Autodesk Inventor part; units mm, degrees
ref_plane "YZ Plane" through (0, 0, 0) normal (1, 0, 0) x (0, 1, 0)
ref_plane "XZ Plane" through (0, 0, 0) normal (0, 1, 0) x (-1, 0, 0)
ref_plane "XY Plane" through (0, 0, 0) normal (0, 0, 1) x (1, 0, 0)
sketch "스케치1" plane through (0, 0, 0) normal (0, 0, 1) x (1, 0, 0)
  line L0 (15, -15) -> (-15, -15)
  line L1 (-15, -15) -> (-15, 15)
  line L2 (-15, 15) -> (15, 15)
  line L3 (15, 15) -> (15, -15)
  line L4 (15, -15) -> (-15, 15) construction
  line L5 (-15, -15) -> (15, 15) construction
  point P0 (0, 0)
  dimension "d0" = 30
  dimension "d1" = 30
extrude "돌출1" add sketch "스케치1" along normal blind 2
sketch "스케치2" plane through (0, 0, 2) normal (0, 0, 1) x (1, 0, 0)
  line L0 (-15, 15) -> (-15, -15)
  line L1 (-15, -15) -> (15, -15)
  line L2 (-15, 15) -> (-12, 15)
  line L3 (-12, 15) -> (-12, -15)
  line L4 (-12, -15) -> (-15, -15)
  line L5 (-15, -15) -> (-15, 15)
  line L6 (15, -15) -> (15, 15)
  line L7 (15, 15) -> (12, 15)
  line L8 (12, 15) -> (12, -15)
  line L9 (12, -15) -> (15, -15)
  line L10 (15, -15) -> (15, 15)
  point P0 (0, 0)
  dimension "d4" = 3
  dimension "d5" = 3
extrude "돌출2" add sketch "스케치2" along normal blind 30
sketch "스케치3" plane through (0, 0, 0) normal (0, 0, -1) x (-1, 0, 0)
  circle A0 centre (0, 0) radius 5
  dimension "d8" = 10
extrude "돌출3" add sketch "스케치3" along normal blind 1
sketch "스케치4" plane through (15, -15, 0) normal (1, 0, 0) x (0, 0, -1)
  line L0 (0, 0) -> (-39, 0)
  line L1 (-39, 0) -> (-26.5, 0)
  line L2 (-2, 0) -> (-32, 0)
  line L3 (-26.5, 0) -> (-26.5, 10)
  circle A0 centre (-26.5, 10) radius 2.5
  line L4 (0, 0) -> (-32, 0)
  line L5 (0, 0) -> (-34, 0)
  line L6 (-34, 0) -> (-21.5, 0)
  line L7 (-21.5, 0) -> (-21.5, 10)
  circle A1 centre (-21.5, 10) radius 2.5
  point P0 (0, 15)
  dimension "d11" = 39
  dimension "d12" = 12.5
  dimension "d13" = 5
  dimension "d14" = 10
  dimension "d32" = 34
  dimension "d33" = 12.5
extrude "돌출4" add sketch "스케치4" against normal blind 12.5 contours A1
sketch "스케치5" plane through (-15, -15, 0) normal (-1, 0, 0) x (0, 0, 1)
  circle A0 centre (26.5, 10) radius 2.5
  circle A1 centre (21.5, 10) radius 2.5
  circle A2 centre (21.5, 10) radius 2.5
  point P0 (0, 15)
extrude "돌출5" add sketch "스케치5" against normal blind 12.5 contours A1
sketch "스케치6" plane through (15, -15, 0) normal (1, 0, 0) x (0, 0, -1)
  line L0 (0, 30) -> (-32, 30)
  line L1 (-2, 30) -> (-32, 30)
  line L2 (-2, 30) -> (-32, 30)
  line L3 (0, 30) -> (-32, 30)
  line L4 (-2, 0) -> (-2, 30)
  line L5 (-2, 30) -> (-2, 0)
  line L6 (0, 30) -> (-32, 30)
  line L7 (-2, 30) -> (-2, 0)
  line L8 (0, 30) -> (-2, 30)
  line L9 (-2, 30) -> (-7, 30)
  line L10 (-2, 30) -> (-32, 30)
  line L11 (-32, 0) -> (-32, 30)
  line L12 (-7, 30) -> (-32, 30)
  line L13 (-32, 30) -> (-32, 20)
  line L14 (-32, 20) -> (-7, 30)
  circle A0 centre (-26.5, 10) radius 2.5
  line L15 (0, 0) -> (-32, 0)
  line L16 (-32, 0) -> (-27, 0)
  line L17 (-27, 0) -> (-27, 22)
  point P0 (0, 15)
  point P1 (-7, 30)
  dimension "d19" = 2
  dimension "d20" = 5
  dimension "d21" = 10
  dimension "d22" = 5
extrude "돌출6" cut sketch "스케치6" against normal through all contours L14 L11 L0 | L17 A0 L15 L11 L14 | L17 A0 picked at (-27.6602, 9.8965)
sketch "스케치7" plane through (15, -15, 0) normal (1, 0, 0) x (0, 0, -1)
  line L0 (-2, 0) -> (-2, 30)
  line L1 (-2, 30) -> (-2, 25)
  line L2 (-2, 30) -> (-2, 0)
  line L3 (-2, 25) -> (-27, 25)
  line L4 (-27, 22) -> (-27, 0)
  arc A0 (-27, 7.5505) -> (-27, 12.4495) centre (-26.5, 10) ccw
  line L5 (-27, 25) -> (-27, 15)
  line L6 (-27, 15) -> (-2, 25)
  line L7 (-27, 22) -> (-27, 0)
  line L8 (0, 0) -> (-27, 0)
  line L9 (0, 0) -> (0, 30)
  line L10 (0, 30) -> (-7, 30)
  line L11 (-7, 30) -> (-27, 22)
  point P0 (0, 15)
  point P1 (-2, 25)
  dimension "d25" = 5
  dimension "d26" = 10
extrude "돌출7" cut sketch "스케치7" against normal through all contours L3 L11 L10 L0 | L6 L4 L11 L3
sketch "스케치8" plane through (15, -15, 0) normal (1, 0, 0) x (0, 0, -1)
  line L0 (0, 0) -> (0, 30)
  line L1 (0, 30) -> (0, 25)
  line L2 (0, 25) -> (-2, 25)
  line L3 (0, 30) -> (-2, 30)
  line L4 (-2, 25) -> (-2, 30)
  line L5 (0, 30) -> (-2, 30)
  point P0 (0, 15)
  dimension "d29" = 5
extrude "돌출8" cut sketch "스케치8" against normal through all
properties part number "castor_link2" material "알루미늄 6061"
Part model, mm, in its own coordinate system. A direction names the side the tool comes from. Coordinates: 2 decimals unless noted, no trailing zeros. Write each loop counter-clockwise with the first axis right and the second up, starting at its lowest first coordinate (ties: lowest second). Pieces come first, ordered by that corner, then holes.
Item 1: Slice it at A-A (z = 21.5). Write the cut outline in (x, y), and give its area (3 significant figures).
Item 2: Slice it at B-B (x = -4). Write the cut outline in (y, z).
Item 3: Probe line 1 (X direction, y = -5, z = 13.25); line 2 (Z direction, x = 10, y = 4); line 3 (Z direction, x = 8.25, y = -7). List the from-to ranges inside material, lowest first.
Item 4: Slice it at D-D (y = -6.25). Write the cut outline in (x, z).
Item 5: Slice it at C-C (x = 0). Write the cut outline in (y, z).
Item 6: Pin check, flat tips, straight feed: pin 1 (1.5 mm diameter, centred on x = -10.5, y = 6.5, fed in from -Z); pin 2 (4 mm diameter, centred on x = -4.5, z = 24, fed in from -Y); pin 3 (1.5 mm diameter, centred on x = -8.5, z = 23.5, fed in from -Y). Stop position of each tip, or through.
Item 7: Which spindle directions (+Z, -Z, +X, -X, +Y, -Y) get a long thin tool onto all of the face, cutting with end or side? Do faces 1 (the face through (-7, -5, 19)), 2 (the face through (-2.5, -5, 21)), 3 (the face through (-13, -8, 27)). Say none if no direction does.
Item 8: Mould opens along X. For faces 4 (the face through (15, -5, 14)), 5 (the face through (1.08, 4.88, -0.49)), 6 (the face through (0, -3, 2)), 7 (the face through (0, 10, 1)) say: released by +X, released by -X, zero draft, split by the parting line, or undercut.
Results found:
1. outline: (-15, -15) - (-12, -15) - (-12, -7.5) - (-2.5, -7.5) - (-2.5, -2.5) - (-12, -2.5) - (-12, 2.2) - (-15, 2.2) - close; (2.5, -7.5) - (12, -7.5) - (12, -15) - (15, -15) - (15, 2.2) - (12, 2.2) - (12, -2.5) - (2.5, -2.5) - close
1. area: 198 mm2
2. outline: (-15, 0) - (-3, 0) - (-3, -1) - (3, -1) - (3, 0) - (10, 0) - (10, 2) - (-15, 2) - close; circle Ø5 at (-5, 21.5)
3. line 1: x = -15 to -12, 12 to 15
3. line 2: z = 0 to 2
3. line 3: z = 0 to 2, 20 to 23
4. outline: (-15, 0) - (15, 0) - (15, 27) - (12, 27) - (12, 23.67) - (2.5, 23.67) - (2.5, 19.33) - (12, 19.33) - (12, 2) - (-12, 2) - (-12, 19.33) - (-2.5, 19.33) - (-2.5, 23.67) - (-12, 23.67) - (-12, 27) - (-15, 27) - close
5. outline: (-15, 0) - (-5, 0) - (-5, -1) - (5, -1) - (5, 0) - (10, 0) - (10, 2) - (-15, 2) - close
6. pin 1: stops at z = 0
6. pin 2: stops at y = -7.45
6. pin 3: stops at y = -7.17
7. face 1: none
7. face 2: +Z, +Y, -Y
7. face 3: +Z, +X, -X, +Y, -Y
8. face 4: released by +X
8. face 5: split by the parting line
8. face 6: undercut
8. face 7: zero draft
